from build123d import *

# Parameters (mm, degrees)
SKETCH006_W     = 100
SKETCH006_H     = 260
PAD001_DEPTH    = 1
POCKET005_DEPTH = 5
FILLET_R        = 10


with BuildPart() as part:
    # Sketch006 → Pad001 (new body)
    with BuildSketch(Plane.XY):
        with Locations((-350, 0)):
            Rectangle(SKETCH006_W, SKETCH006_H)
    extrude(amount=PAD001_DEPTH)

    # Sketch007 (on Face6 of Pad001) → Pocket005 (cut)
    with BuildSketch(Plane.XY.offset(1)):
        with BuildLine():
            ThreePointArc((-347, -80), (-350, -77), (-353, -80))
            Line((-353, -80), (-353, -120))
            ThreePointArc((-353, -120), (-350, -123), (-347, -120))
            Line((-347, -80), (-347, -120))
        make_face()
        with BuildLine():
            ThreePointArc((-387, -80), (-390, -77), (-393, -80))
            Line((-393, -80), (-393, -120))
            ThreePointArc((-393, -120), (-390, -123), (-387, -120))
            Line((-387, -80), (-387, -120))
        make_face()
        with BuildLine():
            ThreePointArc((-307, -80), (-310, -77), (-313, -80))
            Line((-313, -80), (-313, -120))
            ThreePointArc((-313, -120), (-310, -123), (-307, -120))
            Line((-307, -80), (-307, -120))
        make_face()
        with BuildLine():
            ThreePointArc((-347, 120), (-350, 123), (-353, 120))
            Line((-353, 120), (-353, 80))
            ThreePointArc((-353, 80), (-350, 77), (-347, 80))
            Line((-347, 120), (-347, 80))
        make_face()
        with BuildLine():
            ThreePointArc((-387, 120), (-390, 123), (-393, 120))
            Line((-393, 120), (-393, 80))
            ThreePointArc((-393, 80), (-390, 77), (-387, 80))
            Line((-387, 120), (-387, 80))
        make_face()
        with BuildLine():
            ThreePointArc((-307, 120), (-310, 123), (-313, 120))
            Line((-313, 120), (-313, 80))
            ThreePointArc((-313, 80), (-310, 77), (-307, 80))
            Line((-307, 120), (-307, 80))
        make_face()
    extrude(amount=-POCKET005_DEPTH, mode=Mode.SUBTRACT)

    # Fillet
    fillet_edges = [part.edges().sort_by_distance(p)[0] for p in [
        (-400, 130, 0.5),
        (-400, -130, 0.5),
        (-300, -130, 0.5),
        (-300, 130, 0.5),
    ]]
    fillet(fillet_edges, radius=FILLET_R)


solid = part.part
For this review, take the finished solid that the model builds, in its own axes (mm). Coordinates: 2 decimals unless noted, no trailing zeros. Loops run counter-clockwise (first coordinate to the right, second up) from the corner with the lowest first, then second, coordinate; pieces in that order, holes last. Notation, with made-up numbers: (84, -19) -> (133, -19) arc R8 cw to (133, -12) -> close; hole circle Ø6 at (68.5, 55.25). An arc over 180 degrees is marked (long way). Write each question's results on one line, items separated by ' | '.
Q1. To check wall thickness, follow line 1 along X through (y, z) = (90.5, 0.15); line 2 along Y through (x, z) = (-395.5, 0.35). State the ranges of each line that lie inside material, in increasing order. Write a range as [from, to].
Taken from the geometry:
line 1: [-400, -393], [-387, -353], [-347, -313], [-307, -300] | line 2: [-128.35, 128.35]
Q2. Mouldability with a two-part tool opening along Y and no side actions: class faces 1 (the cylindrical face through (-303.01, -127.15, 0.51)), 2 (the flat face through (-351, 2, 1)), 3 (the cylindrical face through (-303.01, 127.15, 0.51)) as +Y half, -Y half, draft (parallel to the pull), parting line (faces both ways), or undercut.
Taken from the geometry:
face 1: -Y half | face 2: draft | face 3: +Y half
Q3. Add section B-B, the plane y = -93. State the section outline as (x, z) points, then the cut area to 3 significant figures.
Taken from the geometry:
outline: (-400, 0) -> (-393, 0) -> (-393, 1) -> (-400, 1) -> close; (-387, 0) -> (-353, 0) -> (-353, 1) -> (-387, 1) -> close; (-347, 0) -> (-313, 0) -> (-313, 1) -> (-347, 1) -> close; (-307, 0) -> (-300, 0) -> (-300, 1) -> (-307, 1) -> close | area: 82.0 mm²
Q4. Add section C-C, the plane z = 0.25. Count the separate pieces of the cut face and the enclosed holes in it, then the cut area to 3 significant figures.
Taken from the geometry:
separate pieces: 1 | enclosed holes: 6 | area: 24,300 mm²
Q5. Add section A-A, the plane x = -350. State the section outline as (y, z) points.
Taken from the geometry:
outline: (-130, 0) -> (-123, 0) -> (-123, 1) -> (-130, 1) -> close; (-77, 0) -> (77, 0) -> (77, 1) -> (-77, 1) -> close; (123, 0) -> (130, 0) -> (130, 1) -> (123, 1) -> close
